Source: CAD feature listing. Evaluate the final solid. Frame: model axes, mm. A direction names the side the tool comes from. Give positions to 0.01 mm unless a question says otherwise; leave off trailing zeros. Loops run counter-clockwise (first coordinate to the right, second up) from the corner with the lowest first, then second, coordinate; pieces in that order, holes last.
```python
from build123d import *
from build123d import SkipClean  # not in build123d's __all__

# Parameters (mm, degrees)
F0_R          = 22.5425
F0_R_2        = 12.7
F1_DEPTH      = 9.8425
F2_R          = 3.175
F3_R          = 3.175
F5_R          = 4.92125
F6_DEPTH      = 50.8
F6_DEPTH_BACK = 3.175


with BuildPart() as f1:
    # F0 (on Front) → F1 (new body)
    with BuildSketch(Plane.XZ):
        Circle(F0_R)
        Circle(F0_R_2, mode=Mode.SUBTRACT)
    extrude(amount=F1_DEPTH)

    # F2
    f2_edges = [f1.edges().sort_by_distance(p)[0] for p in [
        (-22.5425, -9.8425, 0),
        (-22.5425, 0, 0),
    ]]
    fillet(f2_edges, radius=F2_R)

    # F3
    f3_edges = [f1.edges().sort_by_distance(p)[0] for p in [
        (-12.7, -9.8425, 0),
        (-12.7, 0, 0),
    ]]
    fillet(f3_edges, radius=F3_R)

    # F5 (on offset) → F6 (join, two sides)
    with BuildSketch(Plane.XY.offset(19.05)) as f6_sk:
        with Locations((0, -4.92125)):
            Circle(F5_R)
    with SkipClean():  # cleaning this boolean's faces spoils the solid; the shape is the same uncleaned
        extrude(amount=F6_DEPTH)
        extrude(f6_sk.sketch, amount=-F6_DEPTH_BACK)


solid = f1.part
```
(1) Ray query, line 1 along Z through (x, y) = (0, -5.9); line 2 along Z through (x, y) = (3, -9); line 3 along X through (y, z) = (-2.25, -3.5). Return the intervals inside material, ascending.
A:
line 1: z = -22.54 to -12.7, 12.7 to 69.85
line 2: z = -21.31 to -13.39, 13.39 to 21.31
line 3: x = -22.13 to -12.35, 12.35 to 22.13
(2) Section A-A, the plane z = 48. Return the cut outline in (x, y).
A:
outline: circle Ø9.84 at (0, -4.92)
(3) Reachability of faces 4 (the cylindrical face through (4.694, -3.443, 44.255)), 5 (the flat face through (-2, -9.842, 16)) from +Z, -Z, +X, -X, +Y, -Y: full face, straight path, thin tool, end or side. Return the list, or none.
A:
face 4: +Z
face 5: +Z, -Z, +X, -X, -Y
(4) Mould query, pull axis Z, two halves, no side actions, for faces 1 (the flat face through (-2, 0, 16)), 2 (the flat face through (0, -5, 69.85)), 3 (the cylindrical face through (-2.75, -4.9, -12.4)). Classes: pulls with the +Z half, pulls with the -Z half, needs draft (parallel to the pull), parting line crosses it, or undercut.
A:
face 1: needs draft
face 2: pulls with the +Z half
face 3: undercut
(5) First-contact query: pin 1 (1.5 mm diameter, centred on x = -14.5, y = -5.5, fed in from -Z); pin 2 (1.5 mm diameter, centred on y = -5.5, z = 28, fed in from -X); pin 3 (2 mm diameter, centred on x = -6, y = -2, fed in from -Z). Flat tips, straight axial feed; report the tip coordinate or a pass-through.
A:
pin 1: stops at z = -17.86
pin 2: stops at x = -4.92
pin 3: stops at z = -21.88
